Build history of the part. All positions in model axes, mm. Face numbers are marked on the shaded views. A direction names the side the tool comes from. Round coordinates to 2 decimals unless told otherwise and drop trailing zeros. Order: outer loops, then holes, each group sorted by start corner. A loop starts at its lowest first (then second) coordinate and runs counter-clockwise, first axis right, second up. Notation, with made-up numbers: (-7, 18.25) -> (11, 18.25) arc R23 ccw to (11, 53.25) -> close; hole circle Ø9 at (86, -22). An arc over 180 degrees is marked (long way). Write item = value, one per line.
from build123d import *

# Parameters (mm, degrees)
BOSS_EXTRUDE1_DEPTH = 9
FILLET1_R           = 6
FILLET2_R           = 4
BOSS_EXTRUDE2_DEPTH = 18
LPATTERN1_COUNT     = 6
LPATTERN1_PITCH     = 6
CUT_EXTRUDE1_DEPTH  = 145.41368733
SKETCH6_W           = 30.064521177
SKETCH6_H           = 12
CUT_EXTRUDE2_DEPTH  = 10
SKETCH8_R           = 1.75
SKETCH8_R_2         = 1.5
BOSS_EXTRUDE3_DEPTH = 3
SKETCH9_R           = 1.25
CUT_EXTRUDE4_DEPTH  = 1
SKETCH10_R          = 1.25
CUT_EXTRUDE5_DEPTH  = 1
CUT_EXTRUDE6_DEPTH  = 1


with BuildPart() as part:
    # Sketch2 → Boss-Extrude1 (new, symmetric)
    with BuildSketch(Plane(origin=(0, 0, 0), x_dir=(1, 0, 0), z_dir=(0, 1, 0))):
        with BuildLine():
            ThreePointArc((7, -67.928205718), (15.472135955, -68.400341673), (15, -76.872477628))
            Line((15, -76.872477628), (10, -85.532731666))
            Line((10, -85.532731666), (10, -135.532731666))
            Line((10, -135.532731666), (-1, -135.532731666))
            Line((-1, -135.532731666), (-1, -128.532731666))
            Line((-1, -128.532731666), (-18, -86.797721556))
            Line((-18, -86.797721556), (-30.999248866, -86.657975615))
            Line((-30.999248866, -86.657975615), (-30.891751988, -76.658553411))
            Line((-30.891751988, -76.658553411), (-17, -71))
            Line((-17, -71), (-3.134175553, -76.992487891))
            Line((-3.134175553, -76.992487891), (7, -67.928205718))
        make_face()
        Polygon((-17, -71), (-22, -73.036659384), (-48.406582583, -8.20848344), (-25.853959684, 0), align=None)
    extrude(amount=BOSS_EXTRUDE1_DEPTH, both=True)

    # Fillet1
    fillet1_edges = [part.edges().sort_by_distance(p)[0] for p in [
        (-48.406582583, 0, 8.20848344),
        (-25.853959684, 0, 0),
    ]]
    fillet(fillet1_edges, radius=FILLET1_R)

    # Fillet2
    fillet2_edges = [part.edges().sort_by_distance(p)[0] for p in [
        (-1, 0, 135.532731666),
        (-30.999248866, 0, 86.657975615),
        (-30.891751988, 0, 76.658553411),
    ]]
    fillet(fillet2_edges, radius=FILLET2_R)

    # Sketch3 → Boss-Extrude2 (add)
    with BuildSketch(Plane(origin=(0, 9, 0), x_dir=(1, 0, 0), z_dir=(0, 1, 0))):
        Polygon((10, -132.532731666), (10, -128.532731666), (14, -130.532731666), align=None)
    boss_extrude2 = extrude(amount=-BOSS_EXTRUDE2_DEPTH)

    # LPattern1: Boss-Extrude2 ×6
    with Locations(*[(0, 0, -i * LPATTERN1_PITCH) for i in range(1, LPATTERN1_COUNT)]):
        add(boss_extrude2)

    # Sketch5 → Cut-Extrude1 (cut, through all)
    with BuildSketch(Plane(origin=(0, 9, 0), x_dir=(1, 0, 0), z_dir=(0, 1, 0))):
        Polygon((7, -120.532731666), (7, -90.532731666), (-8, -90.532731666), align=None)
    extrude(amount=-CUT_EXTRUDE1_DEPTH, mode=Mode.SUBTRACT)

    # Sketch6 → Cut-Extrude2 (cut)
    with BuildSketch(Plane(origin=(-45.762584731, 0, 18.64055953), x_dir=(0.377236894037746, 0, 0.9261167992088009), z_dir=(-0.9261167992088009, 0, 0.377236894037746))):
        with Locations((98.626824562, 0)):
            Rectangle(SKETCH6_W, SKETCH6_H)
    extrude(amount=-CUT_EXTRUDE2_DEPTH, mode=Mode.SUBTRACT)

    # Sketch8 → Boss-Extrude3 (add)
    with BuildSketch(Plane(origin=(0, 9, 0), x_dir=(1, 0, 0), z_dir=(0, 1, 0))):
        with Locations(Location((-26.956481233, -82.701205484, 0), (0, 0, 270))):
            Circle(SKETCH8_R)
        with Locations(Location((11, -72.400341673, 0), (0, 0, 270))):
            Circle(SKETCH8_R)
        with Locations(Location((-40.499373495, -11.715561331, 0), (0, 0, 270))):
            Circle(SKETCH8_R_2)
    boss_extrude3 = extrude(amount=BOSS_EXTRUDE3_DEPTH)

    # Sketch9 → Cut-Extrude4 (cut)
    with BuildSketch(Plane(origin=(0, 12, 0), x_dir=(1, 0, 0), z_dir=(0, 1, 0))):
        with Locations(Location((-26.956481233, -82.701205484, 0), (0, 0, 270))):
            Circle(SKETCH9_R)
    cut_extrude4 = extrude(amount=-CUT_EXTRUDE4_DEPTH, mode=Mode.SUBTRACT)

    # Sketch10 → Cut-Extrude5 (cut)
    with BuildSketch(Plane(origin=(0, 12, 0), x_dir=(1, 0, 0), z_dir=(0, 1, 0))):
        with Locations(Location((11, -72.400341673, 0), (0, 0, 270))):
            Circle(SKETCH10_R)
    cut_extrude5 = extrude(amount=-CUT_EXTRUDE5_DEPTH, mode=Mode.SUBTRACT)

    # Sketch11 → Cut-Extrude6 (cut)
    with BuildSketch(Plane(origin=(0, 9, 0), x_dir=(1, 0, 0), z_dir=(0, 1, 0))):
        with BuildLine():
            Line((-37.543355443, -17.510445966), (-22, -54.366980008))
            ThreePointArc((-22, -54.366980008), (-22.799244197, -56.331975863), (-24.764240053, -55.532731666))
            Line((-24.764240053, -55.532731666), (-40.307595496, -18.676197624))
            ThreePointArc((-40.307595496, -18.676197624), (-39.508351299, -16.711201768), (-37.543355443, -17.510445966))
        make_face()
    cut_extrude6 = extrude(amount=-CUT_EXTRUDE6_DEPTH, mode=Mode.SUBTRACT)

    # Mirror1: Boss-Extrude3, Cut-Extrude4, Cut-Extrude5, Cut-Extrude6 across plane
    add(boss_extrude3.mirror(Plane.ZX))
    add(cut_extrude4.mirror(Plane.ZX), mode=Mode.SUBTRACT)
    add(cut_extrude5.mirror(Plane.ZX), mode=Mode.SUBTRACT)
    add(cut_extrude6.mirror(Plane.ZX), mode=Mode.SUBTRACT)


solid = part.part
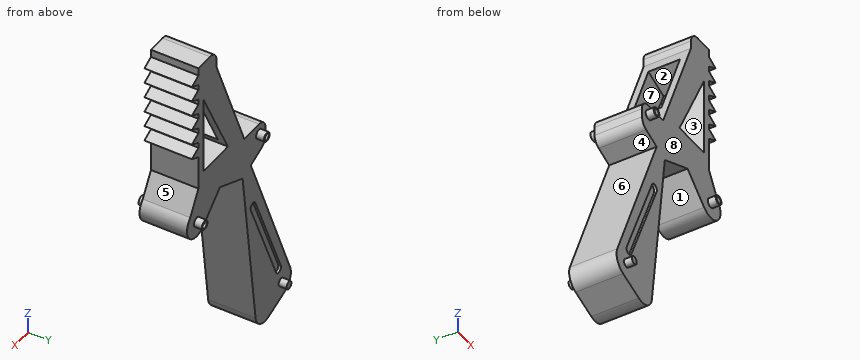
Q1. Flat gauge pins, fed straight in: pin 1 (3 mm diameter, centred on x = -27.5, z = 82, fed in from -Y); pin 2 (1 mm diameter, centred on x = 0.5, z = 112.5, fed in from +Y); pin 3 (12 mm diameter, centred on x = -7.5, z = 96, fed in from -Y); pin 4 (1 mm diameter, centred on y = -5.5, z = 60.5, fed in from -X). Where does each tip first touch, or does it go through?
Check values:
pin_1 = -12
pin_2 = 9
pin_3 = -9
pin_4 = -27.31
Q2. Probe probe 1 along Z at (x, y) = (5, 1.5); probe 2 along Y at (x, z) = (-35, 25); probe 3 along X at (y, z) = (-8.75, 68.5). List the from-to ranges inside material, lowest first.
Check values:
probe_1 = 69.72 to 90.53, 116.53 to 116.75, 120.69 to 135.53
probe_2 = -8 to 8
probe_3 = -23.85 to -17.31, 6.36 to 15.56
Q3. Mould opens along Y. For the marked faces 6, 7 and 8 say: released by +Y, released by -Y, zero draft, split by the parting line, or undercut.
Check values:
face_6 = zero draft
face_7 = undercut
face_8 = released by -Y
Q4. Which spindle directions (+Z, -Z, +X, -X, +Y, -Y) get a long thin tool onto all of the face, cutting with end or side? Do the marked faces 1, 2, 3, 4 and 5. Say none if no direction does.
Check values:
face_1 = -Z, +Y, -Y
face_2 = -X
face_3 = +Y, -Y
face_4 = -X, +Y, -Y
face_5 = +X, +Y, -Y
Q5. Cut at C-C, the plane z = 59. List the corners of the cut face in (x, y).
Check values:
outline = (-27.72, -9) -> (-18.5, -9) -> (-18.5, 9) -> (-27.72, 9) -> close
Q6. Cut at A-A, the plane x = 1. List the corners of the cut face in (y, z), and give its area (3 significant figures).
Check values:
outline = (-9, 73.29) -> (9, 73.29) -> (9, 90.53) -> (-9, 90.53) -> close; (-9, 108.53) -> (-6, 108.53) -> (-6, 122.32) -> (6, 122.32) -> (6, 108.53) -> (9, 108.53) -> (9, 135) -> (-9, 135) -> close
area = 621 mm²
Q7. Cut at B-B, the plane z = 43.5. List the corners of the cut face in (x, y).
Check values:
outline = (-34.03, -9) -> (-29.84, -9) -> (-29.84, -8) -> (-26.58, -8) -> (-26.58, -9) -> (-20.43, -9) -> (-20.43, 9) -> (-26.58, 9) -> (-26.58, 8) -> (-29.84, 8) -> (-29.84, 9) -> (-34.03, 9) -> close
